from build123d import *

# Parameters (mm, degrees)
F0_R          = 9.92251
F1_DEPTH      = 44.45
F2_R          = 8.4181384748
F3_DEPTH      = 7.9385
F4_W          = 73.025
F4_H          = 68.6028956175
F5_DEPTH      = 57.1444816201
F5_DEPTH_BACK = 76.201
F6_R          = 12.7
F7_R          = 4.7625


with BuildPart() as f1:
    # F0 (on Front) → F1 (new body, symmetric)
    with BuildSketch(Plane.XZ):
        with BuildLine():
            Line((0, 44.45), (0, 0))
            Line((0, 0), (133.3434816201, 0))
            Line((133.3434816201, 0), (133.3434816201, 7.9375))
            Line((133.3434816201, 7.9375), (57.1434816201, 7.9375))
            Line((57.1434816201, 7.9375), (57.1434816201, 43.8396862105))
            ThreePointArc((57.1434816201, 43.8396862105), (28.880174299, 73.0233703586), (0, 44.45))
        make_face()
        with Locations((28.575, 44.45)):
            Circle(F0_R, mode=Mode.SUBTRACT)
    extrude(amount=F1_DEPTH, both=True)

    # F2 (on face) → F3 (cut, through all)
    with BuildSketch(Plane.XY.offset(7.9375)):
        with BuildLine():
            ThreePointArc((57.1434816201, 28.575), (59.0033535596, 24.0848719395), (63.4934816201, 22.225))
            Line((63.4934816201, 22.225), (111.1184816201, 22.225))
            ThreePointArc((111.1184816201, 22.225), (126.8339299175, 15.7154481263), (133.3434816201, -2.42e-07))
            Line((133.3434816201, -2.42e-07), (133.3434816201, 44.45))
            Line((133.3434816201, 44.45), (57.1434816201, 44.45))
            Line((57.1434816201, 44.45), (57.1434816201, 36.5125))
            Line((57.1434816201, 36.5125), (57.1434816201, 28.575))
        make_face()
        with BuildLine():
            Line((133.3434816201, -44.45), (133.3434816201, -2.42e-07))
            ThreePointArc((133.3434816201, -2.42e-07), (126.8339297464, -15.7154482974), (111.1184816201, -22.225))
            Line((111.1184816201, -22.225), (63.4934816201, -22.225))
            ThreePointArc((63.4934816201, -22.225), (59.0033535596, -24.0848719395), (57.1434816201, -28.575))
            Line((57.1434816201, -28.575), (57.1434816201, -36.5125))
            Line((57.1434816201, -36.5125), (57.1434816201, -44.45))
            Line((57.1434816201, -44.45), (133.3434816201, -44.45))
        make_face()
        with Locations((73.0184816201, 0)):
            Circle(F2_R)
        with Locations((111.1184816201, 0)):
            Circle(F2_R)
    extrude(amount=-F3_DEPTH, mode=Mode.SUBTRACT)

    # F4 (on face) → F5 (cut, two sides)
    with BuildSketch(Plane.YZ.offset(57.1434816201)) as f5_sk:
        with Locations((0, 42.2389478087)):
            Rectangle(F4_W, F4_H)
    extrude(amount=-F5_DEPTH, mode=Mode.SUBTRACT)
    extrude(f5_sk.sketch, amount=F5_DEPTH_BACK, mode=Mode.SUBTRACT)

    # F6
    f6_edges = [f1.edges().sort_by_distance(p)[0] for p in [
        (28.571741, -44.45, 0),
        (28.571741, 44.45, 0),
    ]]
    fillet(f6_edges, radius=F6_R)

    # F7
    f7_edges = [f1.edges().sort_by_distance(p)[0] for p in [
        (28.571741, 36.5125, 7.9375),
        (28.571741, -36.5125, 7.9375),
    ]]
    fillet(f7_edges, radius=F7_R)


solid = f1.part
Part model, mm, in its own coordinate system. A direction names the side the tool comes from. Coordinates: 2 decimals unless noted, no trailing zeros. Order: outer loops, then holes, each group sorted by start corner. A loop starts at its lowest first (then second) coordinate and runs counter-clockwise, first axis right, second up. Notation, with made-up numbers: M 36.5,79 L 54.5,79 A16 ccw 54.5,100 Z; hole C 75.25,63 d6. An arc over 180 degrees is marked long. Use a Markdown table: item, result.
(1) Cut at C-C on z = 41. Write the cut outline in (x, y).
A:
| item | result |
|---|---|
| outline | M 0,-44.45 L 19.27,-44.45 L 19.27,-36.51 L 0,-36.51 Z; M 0,36.51 L 19.27,36.51 L 19.27,44.45 L 0,44.45 Z; M 37.88,-44.45 L 57.14,-44.45 L 57.14,-36.51 L 37.88,-36.51 Z; M 37.88,36.51 L 57.14,36.51 L 57.14,44.45 L 37.88,44.45 Z |
(2) Flat gauge pins, fed straight in: pin 1 (17.5 mm diameter, centred on y = -34, z = 11, fed in from +X); pin 2 (6.5 mm diameter, centred on x = 85, z = 3, fed in from -Y) (3 decimals); pin 3 (8 mm diameter, centred on y = 35.5, z = 14, fed in from +X). Where does each tip first touch, or does it go through?
A:
| item | result |
|---|---|
| pin 1 | stops at x = 57.78 |
| pin 2 | stops at y = -22.225 |
| pin 3 | stops at x = 57.14 |
(3) Tool access for faces 1 (the flat face through (35, 36.512, 36)), 2 (the cylindrical face through (102.71, 0.37, 4.02)), 3 (the flat face through (57.143, -38, 22)): list every direction of +Z, -Z, +X, -X, +Y, -Y with a clear straight run to the whole face (end or side of a thin tool).
A:
| item | result |
|---|---|
| face 1 | +Z, +X, -X |
| face 2 | +Z, -Z |
| face 3 | +Z, -Z, +X, -Y |
(4) Pull direction X, two halves, no side cores. Call faces 4 (the cylindrical face through (28.172, -35.154, 9.37)), 5 (the cylindrical face through (80.795, -3.224, 4.024)), 6 (the cylindrical face through (58.954, 24.135, 4.024)), 7 (the cylindrical face through (29.51, -40.54, 73.01)): released by +X, released by -X, zero draft, split by the parting line, or undercut.
A:
| item | result |
|---|---|
| face 4 | zero draft |
| face 5 | undercut |
| face 6 | released by +X |
| face 7 | split by the parting line |
(5) Cut at B-B on x = 80. Write the cut outline in (y, z) (1 decimal).
A:
| item | result |
|---|---|
| outline | M -22.2,0 L -4.7,0 L -4.7,7.9 L -22.2,7.9 Z; M 4.7,0 L 22.2,0 L 22.2,7.9 L 4.7,7.9 Z |
(6) Probe L1, parallel to Y at x = 8, z = 41; L2, parallel to X at y = 42, z = 44.45; L3, parallel to Z at x = 8, y = 3. List the from-to ranges inside material, lowest first.
A:
| item | result |
|---|---|
| L1 | y = -44.45 to -36.51, 36.51 to 44.45 |
| L2 | x = 0 to 18.65, 38.5 to 57.15 |
| L3 | z = 0 to 7.94 |
(7) Cut at A-A on z = 11. Write the cut outline in (x, y).
A:
| item | result |
|---|---|
| outline | M 0,-44.34 L 57.14,-44.34 L 57.14,-36.2 L 0,-36.2 Z; M 0,36.2 L 57.14,36.2 L 57.14,44.34 L 0,44.34 Z |
